from build123d import *

# Parameters (mm, degrees)
SKETCH1_W           = 27.4
SKETCH1_H           = 37.4
SKETCH1_W_2         = 5.5
SKETCH1_H_2         = 1
BOSS_EXTRUDE1_DEPTH = 1.5


with BuildPart() as part:
    # Sketch1 → Boss-Extrude1 (new body)
    with BuildSketch(Plane(origin=(0, 0, 0), x_dir=(0, 1, 0), z_dir=(0, 0, 1))):
        Rectangle(SKETCH1_W, SKETCH1_H)
        Rectangle(SKETCH1_W_2, SKETCH1_H_2, mode=Mode.SUBTRACT)
        with Locations((0, 7)):
            Rectangle(SKETCH1_W_2, SKETCH1_H_2, mode=Mode.SUBTRACT)
        with Locations((0, -7)):
            Rectangle(SKETCH1_W_2, SKETCH1_H_2, mode=Mode.SUBTRACT)
    extrude(amount=BOSS_EXTRUDE1_DEPTH)


solid = part.part
Here's how the part is built. I have some questions about the finished solid (model axes, mm). A direction names the side the tool comes from. Coordinates: 2 decimals unless noted, no trailing zeros. Order: outer loops, then holes, each group sorted by start corner. A loop starts at its lowest first (then second) coordinate and runs counter-clockwise, first axis right, second up. Notation, with made-up numbers: M 65,-30 L 84,-30 A15 cw 84,-16 Z; hole C 40,50 d5. An arc over 180 degrees is marked long. Answer as CSV lines item,"result". Start each with the question number.
1. We'd pull the mould along X, two halves only. Please class faces 3 (the flat face through (0, -13.7, 1)), 4 (the flat face through (-6.5, 0, 1)), 5 (the flat face through (18.7, 0, 1)): released by +X, released by -X, zero draft, split by the parting line, or undercut.
2. I want a section at A-A, the plane z = 0.45. Write out the boundary of the cut face in (x, y), and give its area (3 significant figures).
3. I want a section at B-B, the plane y = -2.25. Write out the boundary of the cut face in (x, z).
4. I need wall thicknesses on line 1 (X direction, y = 0.75, z = 0.45). Which ranges of the line are inside material? Lowest first, please. Write a range as [from, to].
5. On a 3-axis mill with a long thin cutter (end or side, diameter ignored), from which of +Z, -Z, +X, -X, +Y, -Y can I reach the whole of each face in a straight line? I mean faces 1 (the flat face through (0, 13.7, 1)), 2 (the flat face through (0.5, 0, 1)). Say none if no direction works.
Recorded:
1,face 3,"zero draft"
1,face 4,"undercut"
1,face 5,"released by +X"
2,outline,"M -18.7,-13.7 L 18.7,-13.7 L 18.7,13.7 L -18.7,13.7 Z; hole M -7.5,-2.75 L -6.5,-2.75 L -6.5,2.75 L -7.5,2.75 Z; hole M -0.5,-2.75 L 0.5,-2.75 L 0.5,2.75 L -0.5,2.75 Z; hole M 6.5,-2.75 L 7.5,-2.75 L 7.5,2.75 L 6.5,2.75 Z"
2,area,"1,010 mm2"
3,outline,"M -18.7,0 L -7.5,0 L -7.5,1.5 L -18.7,1.5 Z; M -6.5,0 L -0.5,0 L -0.5,1.5 L -6.5,1.5 Z; M 0.5,0 L 6.5,0 L 6.5,1.5 L 0.5,1.5 Z; M 7.5,0 L 18.7,0 L 18.7,1.5 L 7.5,1.5 Z"
4,line 1,"x = [-18.7, -7.5], [-6.5, -0.5], [0.5, 6.5], [7.5, 18.7]"
5,face 1,"+Z, -Z, +X, -X, +Y"
5,face 2,"+Z, -Z"
